```python
from build123d import *

# Parameters (mm, degrees)
BOSS_EXTRUDE1_DEPTH   = 16.8
SKETCH1_W             = 4
SKETCH1_H             = 2
BOSS_EXTRUDE1_2_DEPTH = 16.8
SKETCH1_W_2           = 5
BOSS_EXTRUDE1_3_DEPTH = 16.8
SKETCH1_W_3           = 4.8
BOSS_EXTRUDE1_4_DEPTH = 16.8
BOSS_EXTRUDE1_5_DEPTH = 16.8
SKETCH1_3_W           = 100
SKETCH1_3_H           = 30
BOSS_EXTRUDE2_DEPTH   = 2
SKETCH1_6_W           = 10.8
SKETCH1_6_H           = 2
SKETCH1_6_W_2         = 15.2
SKETCH1_6_W_3         = 15.3
BOSS_EXTRUDE4_DEPTH   = 4.6
SKETCH3_W             = 5
SKETCH3_H             = 5
BOSS_EXTRUDE5_DEPTH   = 3
SKETCH4_W             = 11
SKETCH4_H             = 6
CUT_EXTRUDE2_DEPTH    = 4


with BuildPart() as part:
    # Sketch1 → Boss-Extrude1 (new body)
    with BuildSketch(Plane(origin=(0, 0, 0), x_dir=(1, 0, 0), z_dir=(0, 1, 0))):
        Polygon((-87.471226233, -32.96631097), (-87.471226233, -27.96631097), (8.528773767, -27.96631097), (8.528773767, -32.96631097), (8.528773767, -53.96631097), (6.028773767, -53.96631097), (6.028773767, -55.96631097), (10.528773767, -55.96631097), (10.528773767, -25.96631097), (-89.471226233, -25.96631097), (-89.471226233, -55.96631097), (-84.271226233, -55.96631097), (-84.271226233, -53.96631097), (-87.471226233, -53.96631097), (-87.471226233, -48.96631097), align=None)
    extrude(amount=BOSS_EXTRUDE1_DEPTH)



with BuildPart() as body_2:
    # Sketch1 → Boss-Extrude1 2 (new body)
    with BuildSketch(Plane(origin=(0, 0, 0), x_dir=(1, 0, 0), z_dir=(0, 1, 0))):
        with Locations((-71.471226233, -54.96631097)):
            Rectangle(SKETCH1_W, SKETCH1_H)
    extrude(amount=BOSS_EXTRUDE1_2_DEPTH)


with BuildPart() as body_3:
    # Sketch1 → Boss-Extrude1 3 (new body)
    with BuildSketch(Plane(origin=(0, 0, 0), x_dir=(1, 0, 0), z_dir=(0, 1, 0))):
        with Locations((-51.771226233, -54.96631097)):
            Rectangle(SKETCH1_W_2, SKETCH1_H)
    extrude(amount=BOSS_EXTRUDE1_3_DEPTH)


with BuildPart() as body_4:
    # Sketch1 → Boss-Extrude1 4 (new body)
    with BuildSketch(Plane(origin=(0, 0, 0), x_dir=(1, 0, 0), z_dir=(0, 1, 0))):
        with Locations((-31.671226233, -54.96631097)):
            Rectangle(SKETCH1_W_3, SKETCH1_H)
    extrude(amount=BOSS_EXTRUDE1_4_DEPTH)


with BuildPart() as body_5:
    # Sketch1 → Boss-Extrude1 5 (new body)
    with BuildSketch(Plane(origin=(0, 0, 0), x_dir=(1, 0, 0), z_dir=(0, 1, 0))):
        with Locations((-11.671226233, -54.96631097)):
            Rectangle(SKETCH1_W_3, SKETCH1_H)
    extrude(amount=BOSS_EXTRUDE1_5_DEPTH)


with BuildPart() as part_1:
    add(part.part)

    add(body_2.part)  # Boss-Extrude2 merges body 2

    add(body_3.part)  # Boss-Extrude2 merges body 3

    add(body_4.part)  # Boss-Extrude2 merges body 4

    add(body_5.part)  # Boss-Extrude2 merges body 5
    # Sketch1_3 → Boss-Extrude2 (add)
    with BuildSketch(Plane(origin=(0, 0, 0), x_dir=(1, 0, 0), z_dir=(0, 1, 0))):
        with Locations((-39.471226233, -40.96631097)):
            Rectangle(SKETCH1_3_W, SKETCH1_3_H)
    extrude(amount=-BOSS_EXTRUDE2_DEPTH)

    # Sketch1_6 → Boss-Extrude4 (add)
    with BuildSketch(Plane(origin=(0, 0, 0), x_dir=(1, 0, 0), z_dir=(0, 1, 0))):
        with Locations((-78.871226233, -54.96631097)):
            Rectangle(SKETCH1_6_W, SKETCH1_6_H)
        with Locations((-61.871226233, -54.96631097)):
            Rectangle(SKETCH1_6_W_2, SKETCH1_6_H)
        with Locations((-41.671226233, -54.96631097)):
            Rectangle(SKETCH1_6_W_2, SKETCH1_6_H)
        with Locations((-21.671226233, -54.96631097)):
            Rectangle(SKETCH1_6_W_2, SKETCH1_6_H)
        with Locations((-1.621226233, -54.96631097)):
            Rectangle(SKETCH1_6_W_3, SKETCH1_6_H)
    extrude(amount=BOSS_EXTRUDE4_DEPTH)

    # Sketch3 → Boss-Extrude5 (add)
    with BuildSketch(Plane(origin=(0, 0, 0), x_dir=(1, 0, 0), z_dir=(0, 1, 0))):
        with Locations((-84.971226233, -30.46631097)):
            Rectangle(SKETCH3_W, SKETCH3_H)
        with Locations((6.028773767, -30.46631097)):
            Rectangle(SKETCH3_W, SKETCH3_H)
        with Locations((6.028773767, -51.46631097)):
            Rectangle(SKETCH3_W, SKETCH3_H)
        with Locations((-84.971226233, -51.46631097)):
            Rectangle(SKETCH3_W, SKETCH3_H)
    extrude(amount=BOSS_EXTRUDE5_DEPTH)

    # Sketch4 → Cut-Extrude2 (cut)
    with BuildSketch(Plane.ZY.offset(89.471226233)):
        with Locations((34.46631097, 7)):
            Rectangle(SKETCH4_W, SKETCH4_H)
    extrude(amount=-CUT_EXTRUDE2_DEPTH, mode=Mode.SUBTRACT)


solid = part_1.part
```
Work out the finished part from the listing and answer in its coordinate system (mm). A direction names the side the tool comes from. Give positions to 0.01 mm unless a question says otherwise; leave off trailing zeros. Write each loop counter-clockwise with the first axis right and the second up, starting at its lowest first coordinate (ties: lowest second). Pieces come first, ordered by that corner, then holes.
(1) Straight lines are drawn through the part: line 1 (Z direction, x = 6, y = 1.25); line 2 (X direction, y = 2.25, z = 50); line 3 (X direction, y = 14.5, z = 42.5). For each, find the intervals that lie inside material, in ascending order.
Final values:
line 1: z = 25.97 to 32.97, 48.97 to 55.97
line 2: x = -89.47 to -82.47, 3.53 to 10.53
line 3: x = -89.47 to -87.47, 8.53 to 10.53
(2) Flat-ended cylindrical pins translate along their axes: pin 1 Ø5 at (x, y) = (-44.5, 8.5) entering from +Z; pin 2 Ø1.6 at (x, z) = (2, 55) entering from +Y. Find the tip coordinate at first contact, or state that the pin passes through.
Final values:
pin 1: stops at z = 27.97
pin 2: stops at y = 4.6
(3) The mould has two halves that part along Z. Classify faces 6 (the flat face through (3.529, 1, 52)), 7 (the flat face through (-29.271, 11, 55)), 8 (the flat face through (-51, 3, 55.966)): pulls with the +Z half, pulls with the -Z half, needs draft (parallel to the pull), parting line crosses it, or undercut.
Final values:
face 6: undercut
face 7: needs draft
face 8: pulls with the +Z half
(4) The part is cut by section B-B on z = 35. Write down the section's boundary in (x, y), plus the area to 3 significant figures.
Final values:
outline: (-89.47, -2) - (10.53, -2) - (10.53, 16.8) - (8.53, 16.8) - (8.53, 0) - (-87.47, 0) - (-87.47, 4) - (-89.47, 4) - close; (-89.47, 10) - (-87.47, 10) - (-87.47, 16.8) - (-89.47, 16.8) - close
area: 255 mm2
(5) The part is cut by section D-D on x = -28. Write down the section's boundary in (y, z).
Final values:
outline: (-2, 25.97) - (16.8, 25.97) - (16.8, 27.97) - (0, 27.97) - (0, 53.97) - (4.6, 53.97) - (4.6, 55.97) - (-2, 55.97) - close
(6) Which of the six approach directions +Z, -Z, +X, -X, +Y, -Y give full straight-line access (tool end or side, diameter ignored) to faces 1 (the flat face through (-42, 4.6, 55)), 2 (the flat face through (6, 1, 32.966)), 3 (the flat face through (-52, 16.8, 55)), 4 (the flat face through (-88, 4, 34)), 5 (the flat face through (-40, -2, 41))?
Final values:
face 1: +Z, +Y
face 2: +Y
face 3: +Z, -Z, +X, -X, +Y
face 4: -X
face 5: +Z, -Z, +X, -X, -Y
(7) The part is cut by section C-C on y = 11.5. Write down the section's boundary in (x, z).
Final values:
outline: (-89.47, 25.97) - (10.53, 25.97) - (10.53, 55.97) - (6.03, 55.97) - (6.03, 53.97) - (8.53, 53.97) - (8.53, 27.97) - (-87.47, 27.97) - (-87.47, 53.97) - (-84.27, 53.97) - (-84.27, 55.97) - (-89.47, 55.97) - close; (-73.47, 53.97) - (-69.47, 53.97) - (-69.47, 55.97) - (-73.47, 55.97) - close; (-54.27, 53.97) - (-49.27, 53.97) - (-49.27, 55.97) - (-54.27, 55.97) - close; (-34.07, 53.97) - (-29.27, 53.97) - (-29.27, 55.97) - (-34.07, 55.97) - close; (-14.07, 53.97) - (-9.27, 53.97) - (-9.27, 55.97) - (-14.07, 55.97) - close
(8) The part is cut by section A-A on y = 7.75. Count the separate pieces of the cut face and the enclosed holes in it, plus the area to 3 significant figures.
Final values:
separate pieces: 6
enclosed holes: 0
area: 339 mm2
